For this review, take the finished solid that the model builds, in its own axes (mm). A direction names the side the tool comes from. Give positions to 0.01 mm unless a question says otherwise; leave off trailing zeros. Write each loop counter-clockwise with the first axis right and the second up, starting at its lowest first coordinate (ties: lowest second). Pieces come first, ordered by that corner, then holes. Notation, with made-up numbers: (73.5, 20) -> (122.5, 20) arc R26 ccw to (122.5, 36) -> close; hole circle Ø3 at (5, 68.5). An arc over 180 degrees is marked (long way). Write item = value, one per line.
```python
from build123d import *

# Parameters (mm, degrees)
BOSS_EXTRUDE1_DEPTH = 40
SKETCH6_R           = 2.1
CUT_EXTRUDE4_DEPTH  = 12.8
CUT_EXTRUDE7_REACH  = 60.186
SKETCH10_R          = 2.1
SKETCH11_R          = 4.75
CUT_EXTRUDE8_DEPTH  = 4.5
BOSS_EXTRUDE2_START = -0.6
SKETCH12_R          = 2.1
BOSS_EXTRUDE2_DEPTH = 0.6
SKETCH13_W          = 25
SKETCH13_H          = 1.8
BOSS_EXTRUDE3_DEPTH = 1.2
FILLET1_R           = 0.8


with BuildPart() as part:
    # Sketch1 → Boss-Extrude1 (new body)
    with BuildSketch(Plane.XZ):
        Polygon((14, 15.2), (14, 12.8), (14, 11), (39, 11), (39, 12.8), (40.8, 12.8), (40.8, 0), (-40.8, 0), (-40.8, 12.8), (9.2, 12.8), (9.2, 15.2), align=None)
    extrude(amount=BOSS_EXTRUDE1_DEPTH)

    # Sketch6 → Cut-Extrude4 (cut)
    with BuildSketch(Plane(origin=(0, 0, 0), x_dir=(-1, 0, 0), z_dir=(0, 0, -1))):
        with Locations((25, -20)):
            Circle(SKETCH6_R)
        with Locations((0, -20)):
            Circle(SKETCH6_R)
    extrude(amount=-CUT_EXTRUDE4_DEPTH, mode=Mode.SUBTRACT)

    # Sketch10 → Cut-Extrude7 (cut, up to next)
    with BuildSketch(Plane.XY.offset(11), mode=Mode.PRIVATE) as cut_extrude7_sk1:
        with Locations((32.75, -10)):
            Circle(SKETCH10_R)
    cut_extrude7_tool1 = extrude(cut_extrude7_sk1.sketch, amount=-CUT_EXTRUDE7_REACH, mode=Mode.PRIVATE) & part.part
    # Sketch10 → Cut-Extrude7 (cut, up to next)
    with BuildSketch(Plane.XY.offset(11), mode=Mode.PRIVATE) as cut_extrude7_sk2:
        with Locations((32.75, -30)):
            Circle(SKETCH10_R)
    cut_extrude7_tool2 = extrude(cut_extrude7_sk2.sketch, amount=-CUT_EXTRUDE7_REACH, mode=Mode.PRIVATE) & part.part
    add(cut_extrude7_tool1.solids().sort_by_distance((32.75, -10, 11))[0], mode=Mode.SUBTRACT)
    add(cut_extrude7_tool2.solids().sort_by_distance((32.75, -30, 11))[0], mode=Mode.SUBTRACT)

    # Sketch11 → Cut-Extrude8 (cut)
    with BuildSketch(Plane(origin=(0, 0, 0), x_dir=(-1, 0, 0), z_dir=(0, 0, -1))):
        with Locations((-32.75, -10)):
            Circle(SKETCH11_R)
        with Locations((-32.75, -30)):
            Circle(SKETCH11_R)
    extrude(amount=-CUT_EXTRUDE8_DEPTH, mode=Mode.SUBTRACT)

    # Sketch12 → Boss-Extrude2 (add)
    with BuildSketch(Plane(origin=(0, 0, 4.5), x_dir=(-1, 0, 0), z_dir=(0, 0, -1)).offset(BOSS_EXTRUDE2_START)):
        with Locations(Location((-32.75, -10, 0), (0, 0, 180))):
            Circle(SKETCH12_R)
        with Locations(Location((-32.75, -30, 0), (0, 0, 180))):
            Circle(SKETCH12_R)
    extrude(amount=BOSS_EXTRUDE2_DEPTH)

    # Sketch13 → Boss-Extrude3 (add)
    with BuildSketch(Plane.XY.offset(11)):
        with Locations((26.5, -20)):
            Rectangle(SKETCH13_W, SKETCH13_H)
    extrude(amount=BOSS_EXTRUDE3_DEPTH)

    # Fillet1
    fillet1_edges = [part.edges().sort_by_distance(p)[0] for p in [
        (39, 0, 11.9),
        (40.8, 0, 6.4),
        (-40.8, 0, 6.4),
        (9.2, 0, 14),
        (14, 0, 13.1),
        (9.2, -40, 14),
        (-40.8, -40, 6.4),
        (40.8, -40, 6.4),
        (39, -40, 11.9),
        (14, -40, 13.1),
    ]]
    fillet(fillet1_edges, radius=FILLET1_R)


solid = part.part
```
(1) Take a section at A-A (y = -20). Write out the cut boundary in (x, z), plus the area to 3 significant figures.
Answers below:
outline = (-40.8, 0) -> (-27.1, 0) -> (-27.1, 12.8) -> (-40.8, 12.8) -> close; (-22.9, 0) -> (-2.1, 0) -> (-2.1, 12.8) -> (-22.9, 12.8) -> close; (2.1, 0) -> (40.8, 0) -> (40.8, 12.8) -> (39, 12.8) -> (39, 12.2) -> (14, 12.2) -> (14, 15.2) -> (9.2, 15.2) -> (9.2, 12.8) -> (2.1, 12.8) -> close
area = 933 mm^2
(2) Take a section at C-C (x = 32.75). Write out the cut boundary in (y, z), plus the area to 3 significant figures.
Answers below:
outline = (-40, 0) -> (-34.75, 0) -> (-34.75, 4.5) -> (-25.25, 4.5) -> (-25.25, 0) -> (-14.75, 0) -> (-14.75, 4.5) -> (-5.25, 4.5) -> (-5.25, 0) -> (0, 0) -> (0, 11) -> (-7.9, 11) -> (-7.9, 5.1) -> (-12.1, 5.1) -> (-12.1, 11) -> (-19.1, 11) -> (-19.1, 12.2) -> (-20.9, 12.2) -> (-20.9, 11) -> (-27.9, 11) -> (-27.9, 5.1) -> (-32.1, 5.1) -> (-32.1, 11) -> (-40, 11) -> close
area = 307 mm^2
(3) Take a section at D-D (y = -37). Write out the cut boundary in (x, z).
Answers below:
outline = (-40.8, 0) -> (40.8, 0) -> (40.8, 12.8) -> (39, 12.8) -> (39, 11) -> (14, 11) -> (14, 15.2) -> (9.2, 15.2) -> (9.2, 12.8) -> (-40.8, 12.8) -> close
(4) For pin 1 (3.5 mm diameter, centred on x = 32.75, y = -30, fed in from +Z); pin 2 (3.5 mm diameter, centred on x = 32.5, y = -30.5, fed in from +Z); pin 3 (1.5 mm diameter, centred on x = -21, y = -8, fed in from +Z), all flat-tipped, find the tip position at first contact; note any pin that passes through.
Answers below:
pin_1 = 5.1
pin_2 = 11
pin_3 = 12.8
(5) The part is to be moulded in two halves that separate along Y. For faces 1 (the face through (33, -30, 5.1)), 2 (the face through (26, -30, 11)), 3 (the face through (1, -40, 6)), say which applies: released by +Y, released by -Y, zero draft, split by the parting line, or undercut.
Answers below:
face_1 = undercut
face_2 = zero draft
face_3 = released by -Y
(6) To check wall thickness, follow probe 1 along Y at (x, z) = (32.75, 9.5); probe 2 along X at (y, z) = (-24, 12.5); probe 3 along Y at (x, z) = (-25, 3.75). State the ranges of each line that lie inside material, in increasing order.
Answers below:
probe_1 = -40 to -32.1, -27.9 to -12.1, -7.9 to 0
probe_2 = -40.8 to 14, 39 to 40.8
probe_3 = -40 to -22.1, -17.9 to 0
(7) Take a section at B-B (z = 3.25). Write out the cut boundary in (x, y).
Answers below:
outline = (-40.8, -39.2) arc R0.8 ccw to (-40, -40) -> (40, -40) arc R0.8 ccw to (40.8, -39.2) -> (40.8, -0.8) arc R0.8 ccw to (40, 0) -> (-40, 0) arc R0.8 ccw to (-40.8, -0.8) -> close; hole circle Ø4.2 at (-25, -20); hole circle Ø4.2 at (0, -20); hole circle Ø9.5 at (32.75, -30); hole circle Ø9.5 at (32.75, -10)
(8) Tool access review of faces 4 (the face through (30.65, -9.91, 8.09)), 5 (the face through (-16, -20, 12.8)), 6 (the face through (28.362, -31.819, 2.218)): name each direction out of +Z, -Z, +X, -X, +Y, -Y from which nothing blocks a thin tool from reaching the whole face with its end or side.
Answers below:
face_4 = +Z
face_5 = +Z, -X, +Y, -Y
face_6 = -Z
